from build123d import *

# Parameters (mm, degrees)
SKETCH1_W               = 250
SKETCH1_H               = 175
BOSS_EXTRUDE1_DEPTH     = 125
SKETCH2_W               = 240
SKETCH2_H               = 165
CUT_EXTRUDE1_DEPTH      = 120
SKETCH3_W               = 40.1
SKETCH3_H               = 165
CUT_EXTRUDE2_DEPTH      = 198.246672976
SKETCH6_W               = 250
SKETCH6_H               = 175
BOSS_EXTRUDE2_DEPTH     = 5
SKETCH7_W               = 205
SKETCH7_H               = 30
PIANO_PLUG_DEPTH        = 5
ARM_HOLE_REACH          = 199.247
SKETCH8_W               = 50
SKETCH8_H               = 180
BOSS_EXTRUDE8_REACH     = 216.001
SKETCH4_R               = 6
MAIN_SHAFT_HOLE_DEPTH   = 293.884362846
CUT_EXTRUDE8_DEPTH      = 16
CUT_EXTRUDE8_DEPTH_BACK = 33
SKETCH10_R              = 20
BOTTOM_OPEN_DEPTH       = 28
BOTTOM_OPEN_DEPTH_BACK  = 21
SKETCH11_W              = 230
SKETCH11_H              = 155
SKETCH12_W              = 41.033462292
SKETCH12_H              = 5
BOSS_EXTRUDE4_DEPTH     = 233
SKETCH13_W              = 7.5
SKETCH13_H              = 80
BOSS_EXTRUDE5_DEPTH     = 49
SKETCH14_W              = 44.113211518
SKETCH14_H              = 5
BOSS_EXTRUDE6_DEPTH     = 21
FILLET2_R               = 5
SKETCH16_R              = 2.5
SKETCH16_W              = 20
SKETCH16_H              = 42
SERVO_PLUG_HOLE_DEPTH   = 106
SKETCH17_W              = 49.113211518
SKETCH17_H              = 12.164138601
BOSS_EXTRUDE7_DEPTH     = 23
SKETCH19_W              = 10.1
SKETCH19_H              = 5.6
CUT_EXTRUDE9_DEPTH      = 2
SKETCH21_W              = 10.1
SKETCH21_H              = 1.1
CUT_EXTRUDE10_DEPTH     = 10
SKETCH23_W              = 230
SKETCH23_H              = 113.966537708
MAKE_IT_PANEL1_DEPTH    = 5
SKETCH22_W              = 250
SKETCH22_H              = 175
SKETCH22_W_2            = 240
SKETCH22_H_2            = 165
MAKE_IT_PANEL3_DEPTH    = 120
SKETCH24_W              = 240
SKETCH24_H              = 165
CUT_EXTRUDE11_DEPTH     = 5


with BuildPart() as part:
    # Sketch1 → Boss-Extrude1 (new body)
    with BuildSketch(Plane(origin=(0, 0, 0), x_dir=(1, 0, 0), z_dir=(0, 1, 0))):
        Rectangle(SKETCH1_W, SKETCH1_H)
    extrude(amount=-BOSS_EXTRUDE1_DEPTH)

    # Sketch2 → Cut-Extrude1 (cut)
    with BuildSketch(Plane.XZ.offset(125)):
        Rectangle(SKETCH2_W, SKETCH2_H)
    extrude(amount=-CUT_EXTRUDE1_DEPTH, mode=Mode.SUBTRACT)

    # Sketch3 → Cut-Extrude2 (cut, through all)
    with BuildSketch(Plane(origin=(0, 0, 0), x_dir=(1, 0, 0), z_dir=(0, 1, 0))):
        Rectangle(SKETCH3_W, SKETCH3_H)
    extrude(amount=-CUT_EXTRUDE2_DEPTH, mode=Mode.SUBTRACT)

    # Sketch6 → Boss-Extrude2 (add)
    with BuildSketch(Plane.XZ.offset(125)):
        Rectangle(SKETCH6_W, SKETCH6_H)
    extrude(amount=-BOSS_EXTRUDE2_DEPTH)

    # Sketch7 → Piano Plug (cut)
    with BuildSketch(Plane(origin=(0, 0, -87.5), x_dir=(-1, 0, 0), z_dir=(0, 0, -1))):
        with Locations((0, -105)):
            Rectangle(SKETCH7_W, SKETCH7_H)
    extrude(amount=-PIANO_PLUG_DEPTH, mode=Mode.SUBTRACT)

    # Arm Hole: up to this face of the body (flat: up to its plane)
    arm_hole_end = Plane(part.part.faces().sort_by_distance((0, -120, -2.144615385))[0])
    # Sketch8 → Arm Hole (cut, up to the picked face)
    with BuildSketch(Plane(origin=(0, 0, 0), x_dir=(1, 0, 0), z_dir=(0, 1, 0)), mode=Mode.PRIVATE) as arm_hole_sk1:
        with Locations((-0.05, -2.5)):
            Rectangle(SKETCH8_W, SKETCH8_H)
    arm_hole_tool1 = split(extrude(arm_hole_sk1.sketch, amount=-ARM_HOLE_REACH, mode=Mode.PRIVATE), bisect_by=arm_hole_end, keep=Keep.BOTH, mode=Mode.PRIVATE)
    add(arm_hole_tool1.solids().sort_by(Axis((-0.05, 0, 2.5), (0, -1, 0)))[0], mode=Mode.SUBTRACT)

    # Sketch9 → Boss-Extrude8 (add, up to next)
    with BuildSketch(Plane(origin=(-25.05, 0, 0), x_dir=(0, 0, -1), z_dir=(1, 0, 0)), mode=Mode.PRIVATE) as boss_extrude8_sk1:
        Polygon((87.5, 0), (87.5, -90), (82.5, -90), (82.5, -5), (0, -5), (0, 0), align=None)
    boss_extrude8_tool1 = extrude(boss_extrude8_sk1.sketch, amount=BOSS_EXTRUDE8_REACH, mode=Mode.PRIVATE) - part.part
    add(boss_extrude8_tool1.solids().sort_by_distance((-25.05, -45, -86.244761))[0])

    # Sketch4 → Main Shaft Hole (cut, through all)
    with BuildSketch(Plane.ZY.offset(125)):
        with Locations((0, -62.5)):
            Circle(SKETCH4_R)
    extrude(amount=-MAIN_SHAFT_HOLE_DEPTH, mode=Mode.SUBTRACT)

    # Sketch10 → Cut-Extrude8 (cut, two sides: drawn at the far end of the back side and taken through both)
    with BuildSketch(Plane.ZY.offset(125).offset(-CUT_EXTRUDE8_DEPTH_BACK)):
        with Locations((50.8, -62.5)):
            Circle(SKETCH10_R)
    extrude(amount=CUT_EXTRUDE8_DEPTH + CUT_EXTRUDE8_DEPTH_BACK, mode=Mode.SUBTRACT)

    # Sketch11 → Bottom Open (cut, two sides: drawn at the far end of the back side and taken through both)
    with BuildSketch(Plane(origin=(0, -125, 0), x_dir=(-1, 0, 0), z_dir=(0, -1, 0)).offset(-BOTTOM_OPEN_DEPTH_BACK)):
        Rectangle(SKETCH11_W, SKETCH11_H)
    extrude(amount=BOTTOM_OPEN_DEPTH + BOTTOM_OPEN_DEPTH_BACK, mode=Mode.SUBTRACT)

    # Sketch12 → Boss-Extrude4 (add)
    with BuildSketch(Plane(origin=(-115, 0, 0), x_dir=(0, 0, -1), z_dir=(1, 0, 0))):
        with Locations((56.983268854, -122.5)):
            Rectangle(SKETCH12_W, SKETCH12_H)
    extrude(amount=BOSS_EXTRUDE4_DEPTH)

    # Sketch13 → Boss-Extrude5 (add)
    with BuildSketch(Plane(origin=(0, 0, 82.5), x_dir=(-1, 0, 0), z_dir=(0, 0, -1))):
        with Locations((97.75, -80)):
            Rectangle(SKETCH13_W, SKETCH13_H)
    extrude(amount=BOSS_EXTRUDE5_DEPTH)

    # Sketch14 → Boss-Extrude6 (add)
    with BuildSketch(Plane(origin=(-115, 0, 0), x_dir=(0, 0, -1), z_dir=(1, 0, 0))):
        with Locations((-55.443394241, -122.5)):
            Rectangle(SKETCH14_W, SKETCH14_H)
    extrude(amount=BOSS_EXTRUDE6_DEPTH)

    # Fillet2
    # the kernel refuses this fillet: 5 mm, written as the material it adds along each edge
    with BuildSketch(Plane(origin=(-101.5, -120, 33.5), x_dir=(0, 1, 0), z_dir=(1, 0, 0))) as fillet2_piece_1:
        with BuildLine():
            CenterArc((1.057968965, -5), FILLET2_R, 90, 12.215768954)
            Line((0, -0.113211518), (-0.021159379, -0.015475748))
            ThreePointArc((-0.021159379, -0.015475748), (-0.1, -0.056605759), (-0.1, 0))
            Line((-0.1, 0), (0, 0.1))
            Line((0, 0.1), (1.057968965, 0.1))
            Line((1.057968965, 0.1), (1.057968965, 0))
        make_face()
    extrude(amount=7.5)

    # Sketch16 → Servo Plug Hole (cut)
    with BuildSketch(Plane(origin=(0, 0, 0), x_dir=(0, 0, -1), z_dir=(1, 0, 0))):
        with Locations((-45.543439041, -51.74216133)):
            Circle(SKETCH16_R)
        with Locations((-55.793439041, -51.74216133)):
            Circle(SKETCH16_R)
        with Locations((-50.668439041, -75.74216133)):
            Rectangle(SKETCH16_W, SKETCH16_H)
        with Locations((-45.543439041, -99.74216133)):
            Circle(SKETCH16_R)
        with Locations((-55.793439041, -99.74216133)):
            Circle(SKETCH16_R)
    extrude(amount=-SERVO_PLUG_HOLE_DEPTH, mode=Mode.SUBTRACT)

    # Sketch17 → Boss-Extrude7 (add)
    with BuildSketch(Plane.ZY.offset(101.5)):
        with Locations((57.943394241, -113.9179307)):
            Rectangle(SKETCH17_W, SKETCH17_H)
    extrude(amount=BOSS_EXTRUDE7_DEPTH)

    # Sketch19 → Cut-Extrude9 (cut)
    with BuildSketch(Plane(origin=(0, -120, 0), x_dir=(1, 0, 0), z_dir=(0, 1, 0))):
        with Locations((97.45, 49.8)):
            Rectangle(SKETCH19_W, SKETCH19_H)
        with Locations((-97.45, 49.8)):
            Rectangle(SKETCH19_W, SKETCH19_H)
        with Locations((0, 49.8)):
            Rectangle(SKETCH19_W, SKETCH19_H)
    extrude(amount=-CUT_EXTRUDE9_DEPTH, mode=Mode.SUBTRACT)

    # Sketch21 → Cut-Extrude10 (cut)
    with BuildSketch(Plane(origin=(0, 0, -87.5), x_dir=(-1, 0, 0), z_dir=(0, 0, -1))):
        with Locations((-97.45, -124)):
            Rectangle(SKETCH21_W, SKETCH21_H)
        with Locations((97.45, -124)):
            Rectangle(SKETCH21_W, SKETCH21_H)
        with Locations((0, -124)):
            Rectangle(SKETCH21_W, SKETCH21_H)
    extrude(amount=-CUT_EXTRUDE10_DEPTH, mode=Mode.SUBTRACT)

    # Sketch23 → Make it Panel1 (add)
    with BuildSketch(Plane(origin=(0, -120, 0), x_dir=(1, 0, 0), z_dir=(0, 1, 0))):
        with Locations((0, -20.516731146)):
            Rectangle(SKETCH23_W, SKETCH23_H)
    extrude(amount=-MAKE_IT_PANEL1_DEPTH)

    # Sketch22 → Make it Panel3 (cut)
    with BuildSketch(Plane(origin=(0, -120, 0), x_dir=(1, 0, 0), z_dir=(0, 1, 0))):
        Rectangle(SKETCH22_W, SKETCH22_H)
        Rectangle(SKETCH22_W_2, SKETCH22_H_2, mode=Mode.SUBTRACT)
    extrude(amount=MAKE_IT_PANEL3_DEPTH, mode=Mode.SUBTRACT)


with BuildPart() as make_it_panel3_piece_1:
    # of the separate pieces the step leaves, piece 1, a body of its own (make_it_panel3_pieces)
    add(part.part.solids().sort_by_distance((-101.5, -118.942031035, 33.5))[0])


with BuildPart() as make_it_panel3_piece_2:
    # of the separate pieces the step leaves, piece 2, a body of its own (make_it_panel3_pieces)
    add(part.part.solids().sort_by_distance((-25.05, -5, 82.5))[0])

    # Sketch24 → Cut-Extrude11 (cut)
    with BuildSketch(Plane(origin=(0, 0, 0), x_dir=(1, 0, 0), z_dir=(0, 1, 0))):
        Rectangle(SKETCH24_W, SKETCH24_H)
    extrude(amount=-CUT_EXTRUDE11_DEPTH, mode=Mode.SUBTRACT)


solid = make_it_panel3_piece_1.part
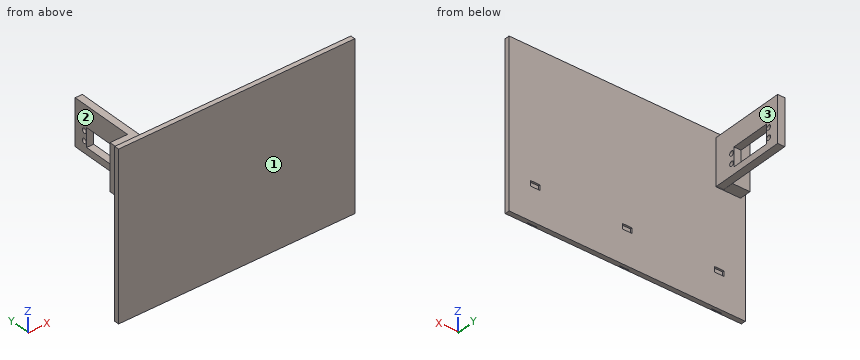
Could you check a few things on this model? Use its own coordinates, in mm. Face numbers are marked on the shaded views. A direction names the side the tool comes from. Coordinates: 2 decimals unless noted, no trailing zeros. Loops run counter-clockwise (first coordinate to the right, second up) from the corner with the lowest first, then second, coordinate; pieces in that order, holes last.
1. Imagine slicing it at D-D (x = 76). Please give me the cut outline in (y, z).
2. Imagine slicing it at B-B (z = 37). Please give me the cut outline in (x, y), and give its area (3 significant figures).
3. I need wall thicknesses on L1, parallel to Y at x = -44, z = -46.5; L2, parallel to X at y = -74, z = 80.5; L3, parallel to Y at x = -114.5, z = 64. Which ranges of each line are inside material? Lowest first, please.
4. For the marked faces 1, 2 and 3, which set-ups out of +Z, -Z, +X, -X, +Y, -Y let a thin tool reach every point of the face, with its end or its side?
5. Imagine slicing it at A-A (y = -81). Please give me the cut outline in (x, z), and give its area (4 significant figures).
6. Imagine slicing it at C-C (y = -111.5). Please give me the cut outline in (x, z).
7. For P1, Ø5, axis at y = -84.5, z = 36, coming from the -X side; P2, Ø8, axis at y = -60, z = 66.5, coming from the +X side; P3, Ø3, axis at x = -1, z = -51, coming from the +Y side, each with a flat end and sliding along its axis, tell me the tip position at first contact or that it passes through.
Computed values:
1. outline: (-125, -87.5) - (-120, -87.5) - (-120, 87.5) - (-125, 87.5) - close
2. outline: (-125, -125) - (125, -125) - (125, -120) - (-94, -120) - (-94, -40) - (-101.5, -40) - (-101.5, -107.84) - (-120, -107.84) - (-120, -120) - (-125, -120) - close
2. area: 2,080 mm2
3. L1: y = -125 to -120
3. L2: x = -101.5 to -94
3. L3: y = -125 to -107.84
4. face 1: +Z, -Z, +X, -X, -Y
4. face 2: +Z, -Z, -X, +Y
4. face 3: +Z, -Z, +X, +Y
5. outline: (-101.5, 33.5) - (-94, 33.5) - (-94, 40.67) - (-101.5, 40.67) - close; (-101.5, 60.67) - (-94, 60.67) - (-94, 82.5) - (-101.5, 82.5) - close
5. area: 217.5 mm2
6. outline: (-120, 33.39) - (-101.5, 33.39) - (-101.5, 33.5) - (-94, 33.5) - (-94, 82.5) - (-120, 82.5) - close
7. P1: stops at x = -101.5
7. P2: stops at x = -94
7. P3: stops at y = -122
